Can you work these out from the model? Positions are in its coordinate system, mm. A direction names the side the tool comes from. Give positions to 0.01 mm unless a question says otherwise; leave off trailing zeros. Order: outer loops, then holes, each group sorted by start corner. A loop starts at its lowest first (then second) coordinate and runs counter-clockwise, first axis right, second up.
Item 1: I want a section at C-C, the plane y = 3.3. Write out the boundary of the cut face in (x, z).
Item 2: I want a section at D-D, the plane x = -7.75. Write out the boundary of the cut face in (y, z) (3 decimals).
Item 3: I want a section at A-A, the plane z = -7. Write out the boundary of the cut face in (x, y).
Item 4: I'm going to push flat-ended pins straight in: pin 1 Ø4 at (x, z) = (-5.5, -11) entering from -Y; pin 2 Ø3 at (x, z) = (-7, 19.5) entering from +Y (3 decimals); pin 3 Ø0.9 at (y, z) = (3.5, -2) entering from +X. Where does each tip first touch, or does it pass through?
Item 5: If I drill on line 1 along Z through (x, y) = (-4.25, 1.9); line 2 along X through (y, z) = (2.3, 7.5); line 3 along Z through (x, y) = (-5.5, 3.2), over which ranges is the centre line in solid material (lowest first)?
Item 6: I want a section at B-B, the plane x = 7.25. Write out the boundary of the cut face in (y, z), then the cut area to 3 significant figures.
Item 7: Which directions (+Z, -Z, +X, -X, +Y, -Y) give clear straight access to the entire face, cutting with the end or side of a thin tool? Please do faces 1 (the flat face through (-3.999, 1.7, 19.5)), 2 (the flat face through (-11, 3, -1)), 3 (the flat face through (11, 3, -1)).
```python
from build123d import *

# Parameters (mm, degrees)
SKETCH1_W       = 24
SKETCH1_H       = 43
PCB_DEPTH       = 1.25
SKETCH2_W       = 22
SKETCH2_H       = 34
RF_CASING_DEPTH = 3
SKETCH5_W       = 6.5
SKETCH5_H       = 3
PINS_DEPTH      = 4


with BuildPart() as part:
    # Sketch1 → PCB (new body)
    with BuildSketch(Plane(origin=(0, 0, 0), x_dir=(1, 0, 0), z_dir=(0, 1, 0))):
        Rectangle(SKETCH1_W, SKETCH1_H)
    extrude(amount=PCB_DEPTH)

    # Sketch2 → RF Casing (add)
    with BuildSketch(Plane(origin=(0, 1.25, 0), x_dir=(1, 0, 0), z_dir=(0, 1, 0))):
        with Locations((0, 1.5)):
            Rectangle(SKETCH2_W, SKETCH2_H)
    extrude(amount=RF_CASING_DEPTH)

    # Sketch5 → Pins (add)
    with BuildSketch(Plane.XY.offset(21.5)):
        with Locations((-7.249153049, 0.625)):
            Rectangle(SKETCH5_W, SKETCH5_H)
    extrude(amount=-PINS_DEPTH)


solid = part.part
```
Results list:
1. outline: (-11, -18.5) - (11, -18.5) - (11, 15.5) - (-11, 15.5) - close
2. outline: (-0.875, 17.5) - (0, 17.5) - (0, -21.5) - (1.25, -21.5) - (1.25, -18.5) - (4.25, -18.5) - (4.25, 15.5) - (1.25, 15.5) - (1.25, 17.5) - (2.125, 17.5) - (2.125, 21.5) - (-0.875, 21.5) - close
3. outline: (-12, 0) - (12, 0) - (12, 1.25) - (11, 1.25) - (11, 4.25) - (-11, 4.25) - (-11, 1.25) - (-12, 1.25) - close
4. pin 1: stops at y = 0
4. pin 2: stops at y = 2.125
4. pin 3: stops at x = 11
5. line 1: z = -18.5 to 15.5, 17.5 to 21.5
5. line 2: x = -11 to 11
5. line 3: z = -18.5 to 15.5
6. outline: (0, -21.5) - (1.25, -21.5) - (1.25, -18.5) - (4.25, -18.5) - (4.25, 15.5) - (1.25, 15.5) - (1.25, 21.5) - (0, 21.5) - close
6. area: 156 mm2
7. face 1: +Z, +X, +Y
7. face 2: +Z, -Z, -X, +Y
7. face 3: +Z, -Z, +X, +Y
